Can you work these out from the model? Positions are in its coordinate system, mm. Give positions to 0.01 mm unless a question says otherwise; leave off trailing zeros. Write each loop counter-clockwise with the first axis right and the second up, starting at its lowest first coordinate (ties: lowest second). Pieces come first, ordered by that corner, then holes.
```python
from build123d import *

# Parameters (mm, degrees)
EXTRUDE_1_DEPTH = 2


with BuildPart() as part:
    # 草图3 → 凸台-拉伸1 (new body)
    with BuildSketch(Plane.XY):
        Polygon((41, 20.009783315), (-32.9, 20.009783315), (-32.9, 80.009783315), (-41, 110.001113679), (-41, 60.009783315), (-41, 20.009783315), (-44, 20.009783315), (-44, 15.009783315), (-41, 15.009783315), (-41, 10.009783315), (-41, 7.009783315), (-41, 5.009783315), (-44, 5.009783315), (-44, 0.009783315), (-41, 0.009783315), (-41, -3.990216685), (-26.5, -3.990216685), (-26.5, 3.009783315), (26.5, 3.009783315), (26.5, -3.990216685), (41, -3.990216685), (41, 0.009783315), (44, 0.009783315), (44, 5.009783315), (41, 5.009783315), (41, 7.009783315), (41, 10.009783315), (41, 15.009783315), (44, 15.009783315), (44, 20.009783315), align=None)
        with BuildLine():
            Line((-37.1, -2.090216685), (-29.9, -2.090216685))
            ThreePointArc((-29.9, -2.090216685), (-29.444365081, -0.990216685), (-29.9, 0.109783315))
            Line((-29.9, 0.109783315), (-37.1, 0.109783315))
            Line((-37.1, 0.109783315), (-37.1, -2.090216685))
        make_face(mode=Mode.SUBTRACT)
        with BuildLine():
            Line((37.1, -2.090216685), (29.9, -2.090216685))
            ThreePointArc((29.9, -2.090216685), (29.444365081, -0.990216685), (29.9, 0.109783315))
            Line((29.9, 0.109783315), (37.1, 0.109783315))
            Line((37.1, 0.109783315), (37.1, -2.090216685))
        make_face(mode=Mode.SUBTRACT)
    extrude(amount=EXTRUDE_1_DEPTH)


solid = part.part
```
1) For pin 1 Ø1 at (x, z) = (7, 1.5) entering from -Y; pin 2 Ø1 at (y, z) = (-1.5, 1) entering from -X; pin 3 Ø0.6 at (x, z) = (-42, 1) entering from +Y, each with a flat end and sliding along its axis, tell me the tip position at first contact or that it passes through.
Values follow:
pin 1: stops at y = 3.01
pin 2: stops at x = -41
pin 3: stops at y = 20.01
2) Please list where these lines run through material, in increasing order: L1, parallel to Y at x = 35.5, z = 1.05; L2, parallel to X at y = 60, z = 1.9; L3, parallel to X at y = 5.5, z = 0.95.
Values follow:
L1: y = -3.99 to -2.09, 0.11 to 20.01
L2: x = -41 to -32.9
L3: x = -41 to 41
3) Suppose I cut it at A-A on z = 1.25. State how many separate pieces and enclosed holes the cut face has, plus the area to 3 significant figures.
Values follow:
separate pieces: 1
enclosed holes: 2
area: 2,230 mm2
4) Suppose I cut it at D-D on x = -13. Write out the boundary of the cut face in (y, z).
Values follow:
outline: (3.01, 0) - (20.01, 0) - (20.01, 2) - (3.01, 2) - close
5) Suppose I cut it at B-B on x = 35.5. Write out the boundary of the cut face in (y, z).
Values follow:
outline: (-3.99, 0) - (-2.09, 0) - (-2.09, 2) - (-3.99, 2) - close; (0.11, 0) - (20.01, 0) - (20.01, 2) - (0.11, 2) - close
6) Suppose I cut it at C-C on y = 33. Write out the boundary of the cut face in (x, z), plus the area to 3 significant figures.
Values follow:
outline: (-41, 0) - (-32.9, 0) - (-32.9, 2) - (-41, 2) - close
area: 16.2 mm2
